```python
from build123d import *

# Parameters (mm, degrees)
SKETCH1_W           = 15
SKETCH1_H           = 15
SKETCH1_R           = 3.2
BOSS_EXTRUDE1_DEPTH = 92
SKETCH4_W           = 40
SKETCH4_H           = 15
SKETCH4_R           = 2.2
BOSS_EXTRUDE2_DEPTH = 5
CUT_EXTRUDE1_DEPTH  = 75


with BuildPart() as part:
    # Sketch1 → Boss-Extrude1 (new body)
    with BuildSketch(Plane.XY):
        with Locations((43.5, 26)):
            Rectangle(SKETCH1_W, SKETCH1_H)
        with Locations((43.5, 26)):
            Circle(SKETCH1_R, mode=Mode.SUBTRACT)
    extrude(amount=BOSS_EXTRUDE1_DEPTH)

    # Sketch4 → Boss-Extrude2 (add)
    with BuildSketch(Plane.XY.offset(92)):
        with Locations((43.5, 26)):
            Rectangle(SKETCH4_W, SKETCH4_H)
        with Locations((58.5, 26)):
            Circle(SKETCH4_R, mode=Mode.SUBTRACT)
        with Locations((28.5, 26)):
            Circle(SKETCH4_R, mode=Mode.SUBTRACT)
    extrude(amount=-BOSS_EXTRUDE2_DEPTH)

    # Sketch3 → Cut-Extrude1 (cut)
    with BuildSketch(Plane.XY.offset(92)):
        Polygon((40.468911087, 20.75), (46.531088913, 20.75), (49.562177826, 26), (46.531088913, 31.25), (40.468911087, 31.25), (37.437822174, 26), align=None)
    extrude(amount=-CUT_EXTRUDE1_DEPTH, mode=Mode.SUBTRACT)


solid = part.part
```
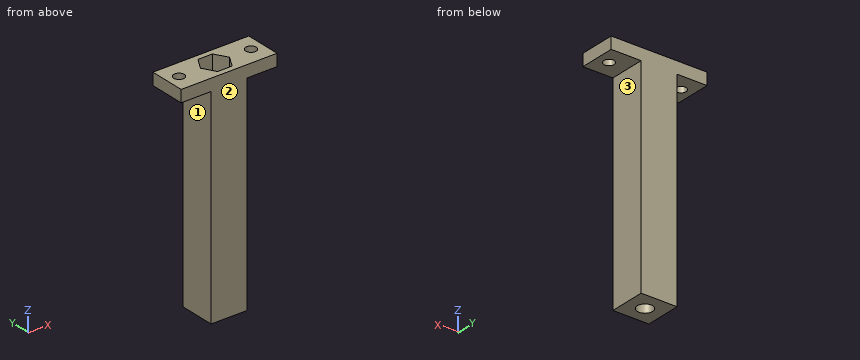
The model under review builds one solid part; all positions refer to its coordinate system, in mm. Face numbers are marked on the shaded views. A direction names the side the tool comes from. Round coordinates to 2 decimals unless told otherwise and drop trailing zeros. Order: outer loops, then holes, each group sorted by start corner. A loop starts at its lowest first (then second) coordinate and runs counter-clockwise, first axis right, second up. Notation, with made-up numbers: (-27.75, 62) - (1.25, 62) arc R25 cw to (1.25, 95) - close; hole circle Ø6 at (61.25, -4.5). An arc over 180 degrees is marked (long way). Answer in a Markdown table with one row per item.
(1) Take a section at C-C on y = 27. Write out the cut boundary in (x, z).
Result set:
| item | result |
|---|---|
| outline | (23.5, 87) - (26.54, 87) - (26.54, 92) - (23.5, 92) - close; (30.46, 87) - (36, 87) - (36, 0) - (40.46, 0) - (40.46, 17) - (38.02, 17) - (38.02, 92) - (30.46, 92) - close; (46.54, 0) - (51, 0) - (51, 87) - (56.54, 87) - (56.54, 92) - (48.98, 92) - (48.98, 17) - (46.54, 17) - close; (60.46, 87) - (63.5, 87) - (63.5, 92) - (60.46, 92) - close |
(2) Take a section at B-B on z = 30.5. Write out the cut boundary in (x, y), plus the area to 3 significant figures.
Result set:
| item | result |
|---|---|
| outline | (36, 18.5) - (51, 18.5) - (51, 33.5) - (36, 33.5) - close; hole (37.44, 26) - (40.47, 20.75) - (46.53, 20.75) - (49.56, 26) - (46.53, 31.25) - (40.47, 31.25) - close |
| area | 130 mm2 |
(3) Take a section at D-D on x = 27.5. Write out the cut boundary in (y, z).
Result set:
| item | result |
|---|---|
| outline | (18.5, 87) - (24.04, 87) - (24.04, 92) - (18.5, 92) - close; (27.96, 87) - (33.5, 87) - (33.5, 92) - (27.96, 92) - close |
(4) For line 1 (Y direction, x = 43.5, z = 12.75); line 2 (Y direction, x = 28.5, z = 88.8); line 3 (X direction, y = 26, z = 7), list the stretches that pass through material, from the lowest coordinate up. Write a range as from..to.
Result set:
| item | result |
|---|---|
| line 1 | y = 18.5..22.8, 29.2..33.5 |
| line 2 | y = 18.5..23.8, 28.2..33.5 |
| line 3 | x = 36..40.3, 46.7..51 |
(5) Machinability: for the marked faces 1, 2 and 3, which of the approach directions +Z, -Z, +X, -X, +Y, -Y give a long, thin tool a straight path to every point of the face, cutting with its end or side? Answer none if there is none.
Result set:
| item | result |
|---|---|
| face 1 | -Z, -X, +Y, -Y |
| face 2 | +Z, -Z, +X, -X, -Y |
| face 3 | -Z, +X, +Y, -Y |
(6) Clearance check with flat-ended pins moving along their axes: P1, Ø6, axis at y = 23.5, z = 30, coming from the +X side; P2, Ø3, axis at x = 43.5, y = 27, coming from the +Z side; P3, Ø7, axis at x = 58.5, y = 26, coming from the -Z side; P4, Ø7.5, axis at x = 43.5, y = 26, coming from the +Z side. State where each tip first meets the part, or that it passes through.
Result set:
| item | result |
|---|---|
| P1 | stops at x = 51 |
| P2 | passes through |
| P3 | stops at z = 87 |
| P4 | stops at z = 17 |
(7) Take a section at A-A on x = 43.5. Write out the cut boundary in (y, z).
Result set:
| item | result |
|---|---|
| outline | (18.5, 0) - (22.8, 0) - (22.8, 17) - (20.75, 17) - (20.75, 92) - (18.5, 92) - close; (29.2, 0) - (33.5, 0) - (33.5, 92) - (31.25, 92) - (31.25, 17) - (29.2, 17) - close |
